For this review, use the dimensioned drawing (mm, ordinates from the lowest corner) and the shaded views. Give positions to 0.01 mm unless a question says otherwise; leave off trailing zeros. Loops run counter-clockwise (first coordinate to the right, second up) from the corner with the lowest first, then second, coordinate; pieces in that order, holes last. Notation, with made-up numbers: M 56.25,5.25 L 83.25,5.25 A25 cw 83.25,39.25 Z; hole C -14,17.25 d2. An arc over 180 degrees is marked long. Return JSON: item names as keys, results as strings.
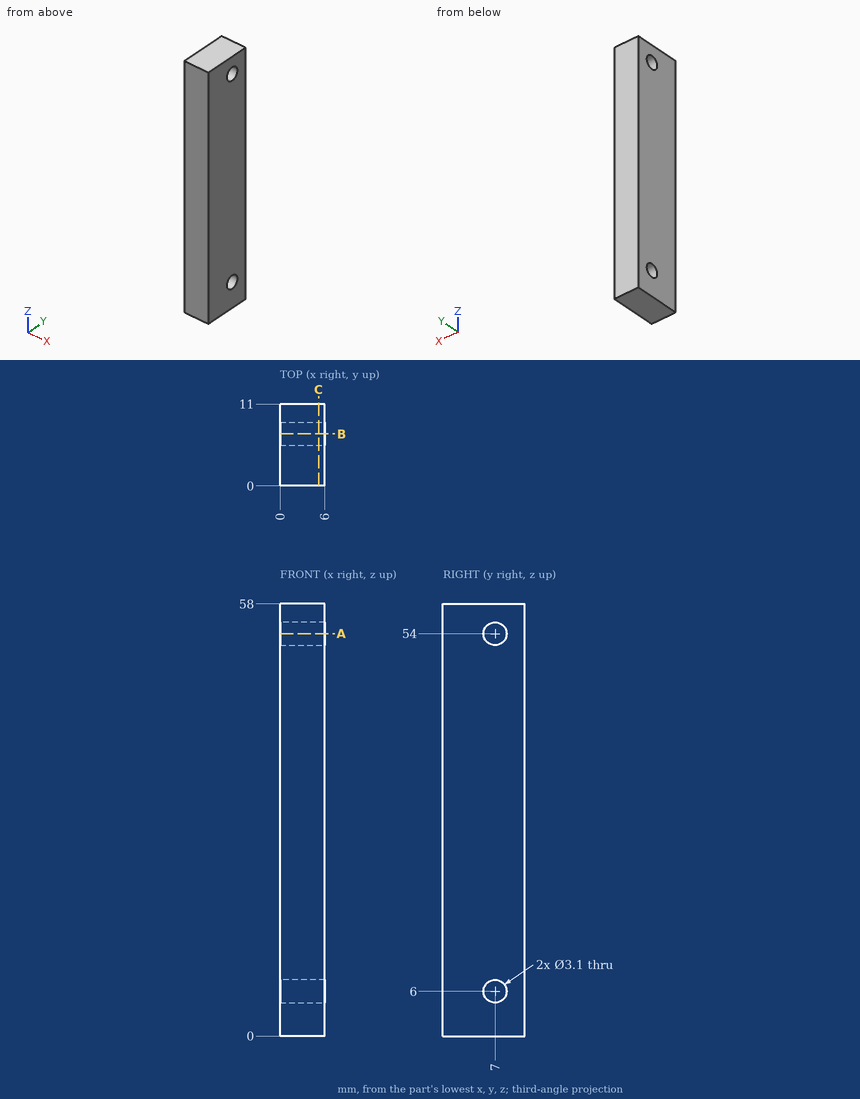
1) Consider section C-C on x = 5.15. Write out the cut boundary in (y, z).
From the geometry:
{"outline": "M 0,0 L 11,0 L 11,58 L 0,58 Z; hole C 7,6 d3.1; hole C 7,54 d3.1"}
2) Wall thickness on L1, parallel to Y at x = 2.75, z = 54; L2, parallel to Z at x = 2.45, y = 6.5: over which ranges is each line inside the solid? List them lowest first. Write a range as from..to.
From the geometry:
{"L1": "0..5.45, 8.55..11", "L2": "0..4.53, 7.47..52.53, 55.47..58"}
3) Consider section A-A on z = 54. Write out the cut boundary in (x, y).
From the geometry:
{"outline": "M 0,0 L 6,0 L 6,5.45 L 0,5.45 Z; M 0,8.55 L 6,8.55 L 6,11 L 0,11 Z"}
4) Insertion check: pin 1 (1 mm diameter, centred on x = 4, z = 15.5, fed in from -Y). The pin has a flat end and moves straight along its axis. Give the tip position at first contact, or say it passes through.
From the geometry:
{"pin 1": "y = 0"}
5) Consider section B-B on y = 7. Write out the cut boundary in (x, z), then the cut area to 3 significant figures.
From the geometry:
{"outline": "M 0,0 L 6,0 L 6,4.45 L 0,4.45 Z; M 0,7.55 L 6,7.55 L 6,52.45 L 0,52.45 Z; M 0,55.55 L 6,55.55 L 6,58 L 0,58 Z", "area": "311 mm²"}
